Design review of the part built by this model. Coordinates are the model's own, in mm. Face numbers are marked on the shaded views. Round coordinates to 2 decimals unless told otherwise and drop trailing zeros. Write each loop counter-clockwise with the first axis right and the second up, starting at its lowest first coordinate (ties: lowest second). Pieces come first, ordered by that corner, then holes. Notation, with made-up numbers: (85.25, 52) -> (120.25, 52) arc R6 ccw to (120.25, 61) -> close; hole circle Ø1 at (36.5, 84). An arc over 180 degrees is marked (long way). Write item = value, one per line. Start each with the question number.
Item 1: Add section A-A, the plane y = -0.5. State the section outline as (x, z) points, then the cut area to 3 significant figures.
Item 2: Mouldability with a two-part tool opening along X and no side actions: class the marked faces 1 and 2 as released by +X, released by -X, zero draft, split by the parting line, or undercut.
Item 3: To check wall thickness, follow L1, parallel to Z at x = -0.5, y = -0.65; L2, parallel to Y at x = -14.5, z = 21; L3, parallel to Z at x = 1, y = 1.1. State the ranges of each line that lie inside material, in increasing order.
Item 4: Add section B-B, the plane z = -8.5. State the section outline as (x, y) points, then the cut area to 3 significant figures.
Item 5: Add section D-D, the plane z = -27. State the section outline as (x, y) points.
Item 6: For pin 1 Ø0.8 at (x, y) = (-16, -0.5) entering from +Z; pin 2 Ø1 at (x, z) = (6.5, 37.5) entering from -Y; pin 3 Ø0.5 at (y, z) = (-0.5, 26) entering from +X, all flat-tipped, find the tip position at first contact; note any pin that passes through.
Item 7: Add section C-C, the plane x = -1.5. State the section outline as (y, z) points.
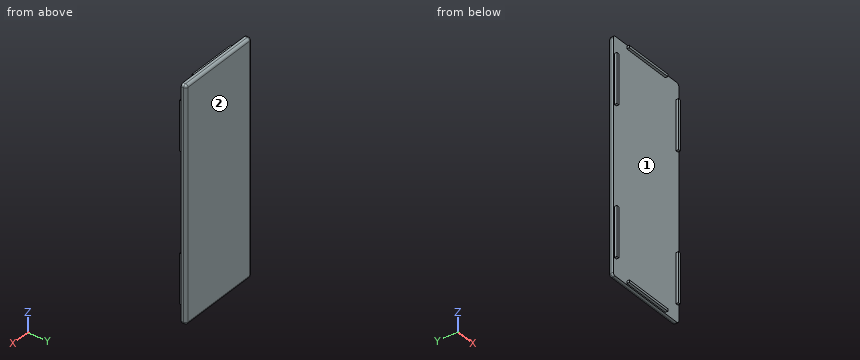
Autodesk Inventor part; units mm, degrees
ref_plane "YZ Plane" through (0, 0, 0) normal (1, 0, 0) x (0, 1, 0)
ref_plane "XZ Plane" through (0, 0, 0) normal (0, 1, 0) x (-1, 0, 0)
ref_plane "XY Plane" through (0, 0, 0) normal (0, 0, 1) x (1, 0, 0)
sketch "Sketch4" plane through (0, 0, 0) normal (0, 1, 0) x (-1, 0, 0)
  line L0 (17, 47) -> (-17, 47)
  line L1 (-17, 47) -> (-17, -47)
  line L2 (-17, -47) -> (17, -47)
  line L3 (17, -47) -> (17, 47)
  line L4 (17, 47) -> (-17, -47) construction
  line L5 (-17, 47) -> (17, -47) construction
  point P0 (0, 0)
  dimension "d52" = 34
  dimension "d53" = 94
extrude "Extrusion5" add sketch "Sketch4" along normal blind 2
sketch "Sketch6" plane through (0, 0, 0) normal (0, -1, 0) x (1, 0, 0)
  line L0 (-16.5, -40) -> (-15.5, -40)
  line L1 (-15.5, -40) -> (-15.5, -20)
  line L2 (-15.5, -20) -> (-16.5, -20)
  line L3 (-16.5, -20) -> (-16.5, -40)
  line L4 (-15.5, 20) -> (-16.5, 20)
  line L5 (-16.5, 20) -> (-16.5, 40)
  line L6 (-16.5, 40) -> (-15.5, 40)
  line L7 (-15.5, 40) -> (-15.5, 20)
  line L8 (-10, 46.5) -> (10, 46.5)
  line L9 (10, 46.5) -> (10, 45.5)
  line L10 (10, 45.5) -> (-10, 45.5)
  line L11 (-10, 45.5) -> (-10, 46.5)
  line L12 (10, 46.5) -> (-10, 46.5)
  line L13 (-10, 46.5) -> (-10, 45.5)
  line L14 (-10, 45.5) -> (10, 45.5)
  line L15 (10, 45.5) -> (10, 46.5)
  line L16 (15.5, 40) -> (16.5, 40)
  line L17 (16.5, 40) -> (16.5, 20)
  line L18 (16.5, 20) -> (15.5, 20)
  line L19 (15.5, 20) -> (15.5, 40)
  line L20 (15.5, -40) -> (16.5, -40)
  line L21 (16.5, -40) -> (16.5, -20)
  line L22 (16.5, -20) -> (15.5, -20)
  line L23 (15.5, -20) -> (15.5, -40)
  line L24 (10, -45.5) -> (-10, -45.5)
  line L25 (-10, -45.5) -> (-10, -46.5)
  line L26 (-10, -46.5) -> (10, -46.5)
  line L27 (10, -46.5) -> (10, -45.5)
  line L28 (-10, -45.5) -> (10, -45.5)
  line L29 (10, -45.5) -> (10, -46.5)
  line L30 (10, -46.5) -> (-10, -46.5)
  line L31 (-10, -46.5) -> (-10, -45.5)
  line L32 (-17, 47) -> (-17, -47)
  line L33 (17, 47) -> (-17, 47)
  line L34 (17, -47) -> (17, 47)
  line L35 (-17, -47) -> (17, -47)
  line L36 (17, 47) -> (17, -47)
  line L37 (-17, -47) -> (-17, 47)
  line L38 (-17, 47) -> (17, 47)
  line L39 (17, -47) -> (-17, -47)
  point P0 (0, 0)
  point P1 (-16, 40)
  point P2 (-16, 20)
  point P3 (16, 40)
  point P4 (16, -40)
  point P5 (-10, -46)
  point P6 (-16, -40)
  dimension "d123" = 1
  dimension "d124" = 20
  dimension "d119" = 1
  dimension "d118" = 20
  dimension "d116" = 20
  dimension "d117" = 1
  dimension "d112" = 20
  dimension "d113" = 1
  dimension "d108" = 1
  dimension "d109" = 20
  dimension "d104" = 1
  dimension "d105" = 20
  dimension "d101" = 20
  dimension "d102" = 1
  dimension "d97" = 20
  dimension "d98" = 1
  dimension "d114" = 7
  dimension "d115" = 0.5
  dimension "d111" = 0.5
  dimension "d110" = 7
  dimension "d107" = 7
  dimension "d106" = 0.5
  dimension "d103" = 0.5
  dimension "d95" = 7
  dimension "d99" = 7
  dimension "d100" = 0.5
  dimension "d96" = 0.5
  dimension "d94" = 7
  dimension "d93" = 7
  dimension "d122" = 0.5
  dimension "d120" = 7
  dimension "d121" = 0.5
  dimension "d133" = 0
  dimension "d134" = 0
  dimension "d135" = 0
  dimension "d136" = 0
extrude "Extrusion7" add sketch "Sketch6" along normal blind 1 contours L3 L2 L1 L0 | L4 L5 L6 L7 | L8 L9 L10 L11 | L16 L17 L18 L19 | L23 L22 L21 L20 | L27 L26 L25 L24
fillet "Fillet9" radius 1 1 edges at (17, 1, -47)
fillet "Fillet10" radius 1 1 edges at (-17, 1, -47)
fillet "Fillet11" radius 1 1 edges at (-17, 1, 47)
fillet "Fillet12" radius 1 1 edges at (17, 1, 47)
fillet "Fillet13" radius 1 8 edges at (-16.7071, 2, -46.7071) (-17, 2, 0) (-16.7071, 2, 46.7071) (0, 2, 47) (16.7071, 2, 46.7071) (17, 2, 0) (16.7071, 2, -46.7071) (0, 2, -47)
properties part number "block_main" material "PC/ABS Plastic"
Result set:
q1.outline = (-16.5, -40) -> (-15.5, -40) -> (-15.5, -20) -> (-16.5, -20) -> close; (-16.5, 20) -> (-15.5, 20) -> (-15.5, 40) -> (-16.5, 40) -> close; (-10, -46.5) -> (10, -46.5) -> (10, -45.5) -> (-10, -45.5) -> close; (-10, 45.5) -> (10, 45.5) -> (10, 46.5) -> (-10, 46.5) -> close; (15.5, -40) -> (16.5, -40) -> (16.5, -20) -> (15.5, -20) -> close; (15.5, 20) -> (16.5, 20) -> (16.5, 40) -> (15.5, 40) -> close
q1.area = 120 mm²
q2.face_1 = undercut
q2.face_2 = zero draft
q3.L1 = -46.5 to -45.5, 45.5 to 46.5
q3.L2 = 0 to 2
q3.L3 = -46.99 to 46.99
q4.outline = (-17, 0) -> (17, 0) -> (17, 1) arc R1 ccw to (16, 2) -> (-16, 2) arc R1 ccw to (-17, 1) -> close
q4.area = 67.6 mm²
q5.outline = (-17, 0) -> (-16.5, 0) -> (-16.5, -1) -> (-15.5, -1) -> (-15.5, 0) -> (15.5, 0) -> (15.5, -1) -> (16.5, -1) -> (16.5, 0) -> (17, 0) -> (17, 1) arc R1 ccw to (16, 2) -> (-16, 2) arc R1 ccw to (-17, 1) -> close
q6.pin_1 = 40
q6.pin_2 = 0
q6.pin_3 = 16.5
q7.outline = (-1, -46.5) -> (0, -46.5) -> (0, -47) -> (1, -47) arc R1 ccw to (2, -46) -> (2, 46) arc R1 ccw to (1, 47) -> (0, 47) -> (0, 46.5) -> (-1, 46.5) -> (-1, 45.5) -> (0, 45.5) -> (0, -45.5) -> (-1, -45.5) -> close
